Check sheet for the modelled part. Datum: model origin and axes. Units: mm. Face numbers are marked on the shaded views. A direction names the side the tool comes from. Coordinates: 2 decimals unless noted, no trailing zeros. Answer in a Markdown table with one row per item. Add a question column.
```python
from build123d import *
from build123d.topology import SkipClean

# Parameters (mm, degrees)
ESQUISSE2_R             = 25
ENL_V_MAT_EXTRU_1_DEPTH = 512.908194894
ESQUISSE3_W             = 16
ESQUISSE3_H             = 8.6
ENL_V_MAT_EXTRU_2_DEPTH = 512.908194894
ECHELLE1_SCALE          = 0.5


with BuildPart() as part:
    # Esquisse1 → Révolution1 (revolve)
    with BuildSketch(Plane(origin=(0, 0, 0), x_dir=(0, 0, -1), z_dir=(1, 0, 0)), mode=Mode.PRIVATE) as r_volution1_sk:
        with BuildLine():
            Line((0, 0), (-50, 0))
            Line((-50, 0), (-50, 75))
            Line((-50, 75), (-25, 104.793839815))
            Line((-25, 104.793839815), (-25, 280.358983849))
            Line((-25, 280.358983849), (-45, 315))
            Line((-45, 315), (-45, 355))
            Line((-45, 355), (-18.820962226, 355))
            Line((-18.820962226, 355), (-9.700735091, 332.98182396))
            ThreePointArc((-9.700735091, 332.98182396), (-5.833487447, 328.269569071), (0, 326.5))
            Line((0, 326.5), (0, 0))
        make_face()
    r_volution1 = revolve(r_volution1_sk.sketch.rotate(Axis((0, 0, 0), (0, 0, 1)), 90), axis=Axis((0, 0, 0), (0, 0, 1)))

    # Symétrie1: Révolution1 across plane
    with SkipClean():  # the faces are left unmerged after this step: merging them gives an invalid solid
        add(r_volution1.mirror(Plane(origin=(0, 326.5, 0), x_dir=(1, 0, 0), z_dir=(0, 0, -1))))

    # Esquisse2 → Enlèv. mat.-Extru.1 (cut, through all)
    with SkipClean():  # the faces are left unmerged after this step: merging them gives an invalid solid
        with BuildSketch(Plane.XY.offset(50)):
            Circle(ESQUISSE2_R)
        extrude(amount=-ENL_V_MAT_EXTRU_1_DEPTH, mode=Mode.SUBTRACT)

    # Esquisse3 → Enlèv. mat.-Extru.2 (cut, through all)
    with SkipClean():  # the faces are left unmerged after this step: merging them gives an invalid solid
        with BuildSketch(Plane.XY.offset(50)):
            with Locations((0, 25)):
                Rectangle(ESQUISSE3_W, ESQUISSE3_H)
        extrude(amount=-ENL_V_MAT_EXTRU_2_DEPTH, mode=Mode.SUBTRACT)


with BuildPart() as part_1:
    # Echelle1: scaled about (0, -0.00849014, 0)
    add(part.part.scale(ECHELLE1_SCALE).moved(Location((0, -0.00424507, 0))))


solid = part_1.part
```
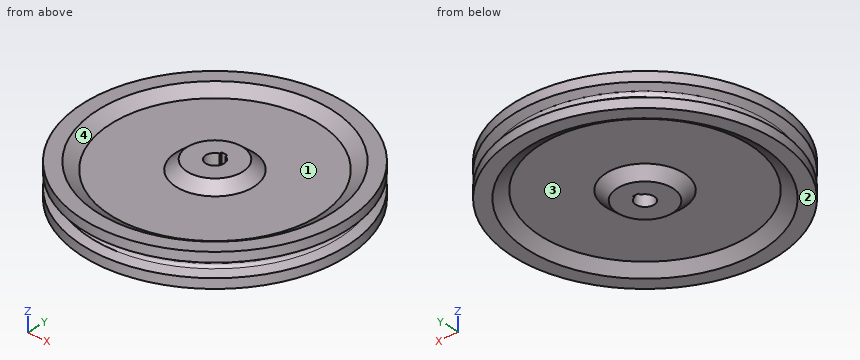
Q1. Access from +Z, -Z, +X, -X, +Y, -Y to the whole of each face (thin tool, end or side, straight path). Record for the marked faces 3 and 4.
Q2. Thickness scan on L1, parallel to Y at x = 0, z = -13.5; L2, parallel to Y at x = 0, z = 11; L3, parallel to Y at x = -18.5, z = -16.5. Record the ranges inside material, lowest first.
Q3. Go/stop test with flat-tipped pins: pin 1 (8 mm diameter, centred on y = -101.5, z = 6.5, fed in from +X); pin 2 (1 mm diameter, centred on x = 136.5, y = -3.5, fed in from -Z); pin 3 (2 mm diameter, centred on y = 13.5, z = -4.5, fed in from -X). Record where each tip stops, or that it passes through.
Q4. Mould release check, pull along X, two halves, no side actions. Record for the marked faces 1 and 2: released by +X, released by -X, zero draft, split by the parting line, or undercut.
Answer key:
| question | item | result |
|---|---|---|
| 1 | face 3 | -Z |
| 1 | face 4 | +Z |
| 2 | L1 | -177.5 to -141.92, -51.21 to -12.5, 14.65 to 51.2, 141.91 to 177.5 |
| 2 | L2 | -177.5 to -12.5, 14.65 to 177.5 |
| 2 | L3 | -176.54 to -145.94, -43.89 to 43.89, 145.94 to 176.53 |
| 3 | pin 1 | x = 147.49 |
| 3 | pin 2 | z = -12.5 |
| 3 | pin 3 | x = -167.52 |
| 4 | face 1 | undercut |
| 4 | face 2 | zero draft |
